Part model, mm, in its own coordinate system. Coordinates: 2 decimals unless noted, no trailing zeros. Write each loop counter-clockwise with the first axis right and the second up, starting at its lowest first coordinate (ties: lowest second). Pieces come first, ordered by that corner, then holes. Notation, with made-up numbers: (49.5, 21.25) - (88.5, 21.25) arc R28 ccw to (88.5, 46.25) - close; hole circle Ø4 at (58.25, 59.5). An arc over 180 degrees is marked (long way). Use a Markdown table: item, result.
Autodesk Inventor part; units mm, degrees
ref_plane "YZ Plane" through (0, 0, 0) normal (1, 0, 0) x (0, 1, 0)
ref_plane "XZ Plane" through (0, 0, 0) normal (0, 1, 0) x (-1, 0, 0)
ref_plane "XY Plane" through (0, 0, 0) normal (0, 0, 1) x (1, 0, 0)
sketch "Sketch1" plane through (0, 0, 0) normal (1, 0, 0) x (0, 1, 0)
  circle A0 centre (0, 0) radius 3.175
  line L0 (3.175, 0) -> (15.875, 0)
  line L1 (15.875, 0) -> (15.875, 11.0604)
  dimension "d0" = 6.35
  dimension "d1" = 12.7
revolve "Revolution1" add sketch "Sketch1" angle 335 about axis through (0, 15.875, 0) along (0, 0, 1)
sketch "Sketch2" plane through (0, 0, 0) normal (0, 1, 0) x (-1, 0, 0)
  circle A0 centre (0, 0) radius 3.175
  line L0 (15.875, -3.175) -> (-15.875, -3.175)
extrude "Extrusion1" add sketch "Sketch2" against normal blind 101.6
sketch "Sketch3" plane through (0, 0, 0) normal (0, 1, 0) x (1, 0, 0)
  line L0 (0, 3.175) -> (0, -3.175)
  arc A0 (0, 3.175) -> (0, -3.175) centre (0, 0) ccw
revolve "Revolution2" add sketch "Sketch3" angle 360 about axis through (0, 0, -3.175) along (0, 0, 1)
fillet "Fillet1" radius 3.175 1 edges at (3.175, -2.9086, 0)
thread "Thread1"
properties part number "EyeBolt"
Item 1: Drill centre lines: probe 1 along Z at (x, y) = (15.5, 15.5); probe 2 along Y at (x, z) = (6.5, -2.5); probe 3 along Y at (x, z) = (-7.5, 0.5). Where is each one in solid material? Low to high.
From the geometry:
| item | result |
|---|---|
| probe 1 | -3.15 to 3.15 |
| probe 2 | -0.73 to 3.57, 28.18 to 32.48 |
| probe 3 | -0.21 to 5.58, 26.17 to 33.34 |
Item 2: Drop flat-ended pins along their axis: P1, Ø2, axis at y = -74, z = 1.5, coming from the +X side; P2, Ø3, axis at x = 13, y = 10.5, coming from the -Z side. Give the stop position or say it passes through.
From the geometry:
| item | result |
|---|---|
| P1 | x = 3.14 |
| P2 | z = -3.16 |
Item 3: Two-plate mould, pull along X, no slides. Class faces 1 (the face through (0, -101.6, 0)), 2 (the face through (-6.728, 1.447, 0.044)): pulls with the +X half, pulls with the -X half, needs draft (parallel to the pull), parting line crosses it, or undercut.
From the geometry:
| item | result |
|---|---|
| face 1 | needs draft |
| face 2 | undercut |
Item 4: Band-saw the part on A-A, the plane y = -47. Give the cut face in (x, z) (3 decimals), then the cut area to 3 significant figures.
From the geometry:
| item | result |
|---|---|
| outline | circle Ø6.35 at (0, 0) |
| area | 31.7 mm^2 |
